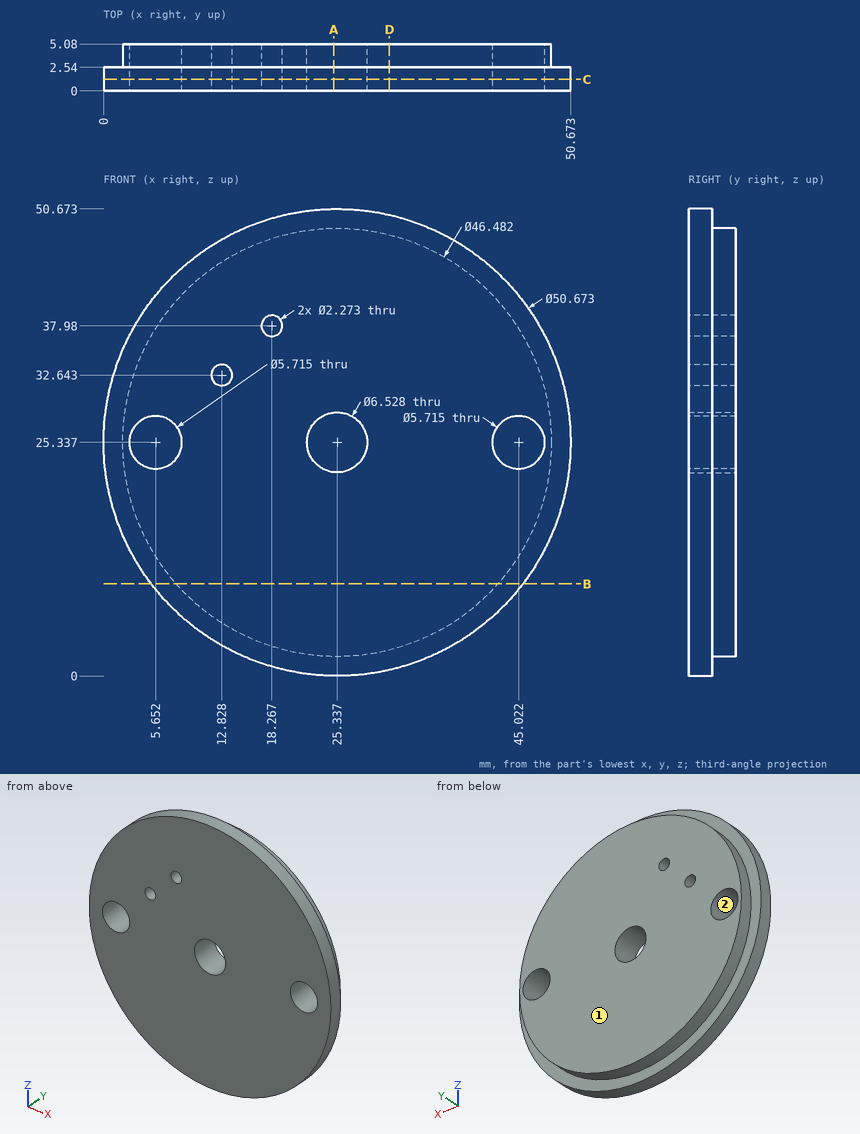
The figure shows three views and two pictorial views of one solid part (mm, origin at its lowest corner). Answer the questions. Coordinates: 2 decimals unless noted, no trailing zeros. Loops run counter-clockwise (first coordinate to the right, second up) from the corner with the lowest first, then second, coordinate; pieces in that order, holes last. Notation, with made-up numbers: (-28.75, 29.25) -> (-22.75, 29.25) arc R20 ccw to (-22.75, 33.25) -> close; hole circle Ø3 at (-29, 1.5). An arc over 180 degrees is marked (long way). Return JSON: item names as keys, results as strings. Group by question number.
(1) A cutting plane is placed at A-A on x = 25. Write down the section's boundary in (y, z) (1 decimal), and give its area (3 significant figures).
(2) Determine the mould class of the marked faces 1 and 2 for opening direction Z: released by +Z, released by -Z, zero draft, split by the parting line, or undercut.
(3) A cutting plane is placed at C-C on y = 1.25. Write down the section's boundary in (x, z) (1 decimal).
(4) A cutting plane is placed at D-D on x = 31. Write down the section's boundary in (y, z), and give its area (3 significant figures).
(5) Given pin 1 Ø1.4 at (x, z) = (12.83, 32.64) entering from +Y; pin 2 Ø3.5 at (x, z) = (18.27, 37.98) entering from -Y; pin 3 Ø2 at (y, z) = (4.5, 8.5) entering from -X (1 decimal), each flat-ended and moving along its own axis, determine where each tip first touches the part or whether it passes through.
(6) A cutting plane is placed at B-B on z = 10. Write down the section's boundary in (x, y) (1 decimal), and give its area (3 significant figures).
(7) Find the intervals of material crossed by probe 1 along Y at (x, z) = (3, 35.5); probe 2 along X at (y, z) = (4.95, 33.5) (1 decimal); probe 3 along Z at (x, y) = (43.5, 3.15) (1 decimal), in increasing order. Write a range as from..to.
The answers:
{
 "1": {"outline": "(0, 0) -> (2.5, 0) -> (2.5, 2.1) -> (5.1, 2.1) -> (5.1, 22.1) -> (0, 22.1) -> close; (0, 28.6) -> (5.1, 28.6) -> (5.1, 48.6) -> (2.5, 48.6) -> (2.5, 50.7) -> (0, 50.7) -> close", "area": "214 mm^2"},
 "2": {"face 1": "zero draft", "face 2": "undercut"},
 "3": {"outline": "circle Ø50.7 at (25.3, 25.3); hole circle Ø5.7 at (5.7, 25.3); hole circle Ø2.3 at (12.8, 32.6); hole circle Ø2.3 at (18.3, 38); hole circle Ø6.5 at (25.3, 25.3); hole circle Ø5.7 at (45, 25.3)"},
 "4": {"outline": "(0, 0.64) -> (2.54, 0.64) -> (2.54, 2.8) -> (5.08, 2.8) -> (5.08, 47.88) -> (2.54, 47.88) -> (2.54, 50.03) -> (0, 50.03) -> close", "area": "240 mm^2"},
 "5": {"pin 1": "passes through", "pin 2": "stops at y = 0", "pin 3": "stops at x = 8.3"},
 "6": {"outline": "(5.2, 0) -> (45.5, 0) -> (45.5, 2.5) -> (42.8, 2.5) -> (42.8, 5.1) -> (7.9, 5.1) -> (7.9, 2.5) -> (5.2, 2.5) -> close", "area": "191 mm^2"},
 "7": {"probe 1": "y = 0..2.54", "probe 2": "x = 3.6..12.1, 13.6..47.1", "probe 3": "z = 10.8..22.9, 27.8..39.8"}
}
